Autodesk Inventor part; units mm, degrees
ref_plane "YZ Plane" through (0, 0, 0) normal (1, 0, 0) x (0, 1, 0)
ref_plane "XZ Plane" through (0, 0, 0) normal (0, 1, 0) x (-1, 0, 0)
ref_plane "XY Plane" through (0, 0, 0) normal (0, 0, 1) x (1, 0, 0)
sketch "스케치1" plane through (0, 0, 0) normal (0, 0, 1) x (1, 0, 0)
  line L0 (-350, 74) -> (350, 74)
  line L1 (350, 74) -> (350, -74)
  line L2 (350, -74) -> (-350, -74)
  line L3 (-350, -74) -> (-350, 74)
  line L4 (-340, 64.5) -> (-211.5, 64.5)
  line L5 (-211.5, 64.5) -> (-211.5, -64)
  line L6 (-211.5, -64) -> (-340, -64)
  line L7 (-340, -64) -> (-340, 64.5)
  line L8 (-201.5, 65) -> (-72.5, 65)
  line L9 (-72.5, 65) -> (-72.5, -64)
  line L10 (-72.5, -64) -> (-201.5, -64)
  line L11 (-201.5, -64) -> (-201.5, 65)
  line L12 (211, 65) -> (340, 65)
  line L13 (340, 65) -> (340, -64)
  line L14 (340, -64) -> (211, -64)
  line L15 (211, -64) -> (211, 65)
  line L16 (72.5, 64.5) -> (201, 64.5)
  line L17 (201, 64.5) -> (201, -64)
  line L18 (201, -64) -> (72.5, -64)
  line L19 (72.5, -64) -> (72.5, 64.5)
  circle A0 centre (0, 0) radius 50
  circle A1 centre (42.072, 42.072) radius 2
  circle A2 centre (-42.072, 42.072) radius 2
  circle A3 centre (-42.072, -42.072) radius 2
  circle A4 centre (42.072, -42.072) radius 2
  line L20 (-490, 0) -> (490, 0)
  line L21 (0, -103.6) -> (0, 103.6)
  point P0 (0, -74)
  point P1 (-72.5, 0.5)
  point P2 (-201.5, 0.5)
  point P3 (-137, -64)
  point P4 (-137, 65)
  point P5 (340, 0.5)
  point P6 (211, 0.5)
  point P7 (275.5, -64)
  point P8 (275.5, 65)
  point P9 (136.75, -64)
  point P10 (136.75, 64.5)
  point P11 (201, 0.25)
  point P12 (72.5, 0.25)
  dimension "d0" = 148
  dimension "d1" = 74
  dimension "d2" = 700
  dimension "d3" = 350
  dimension "d4" = 128.5
  dimension "d5" = 128.5
  dimension "d6" = 10
  dimension "d7" = 10
  dimension "d8" = 129
  dimension "d9" = 129
  dimension "d10" = 10
  dimension "d11" = 10
  dimension "d12" = 129
  dimension "d13" = 129
  dimension "d14" = 128.5
  dimension "d15" = 128.5
  dimension "d16" = 10
  dimension "d17" = 10
  dimension "d18" = 10
  dimension "d19" = 10
  dimension "d20" = 100
  dimension "d21" = 4
  dimension "d22" = 4
  dimension "d23" = 4
  dimension "d24" = 4
  dimension "d25" = 42.072
  dimension "d26" = 42.072
  dimension "d27" = 42.072
  dimension "d28" = 42.072
  dimension "d29" = 42.072
  dimension "d30" = 42.072
  dimension "d31" = 42.072
  dimension "d32" = 42.072
extrude "돌출3" add sketch "스케치1" along normal blind 2 contours L0 L21 A0 L20 L9 L8 L11 L5 L4 L7 L3 | L0 L1 L20 L13 L12 L15 L17 L16 L19 A0 L21 | L20 L7 L6 L5 L11 L10 L9 A0 L21 L2 L3 | L1 L2 L21 A0 L20 L19 L18 L17 L15 L14 L13
properties part number "가로로만"
Can you work these out from the model? Positions are in its coordinate system, mm. Coordinates: 2 decimals unless noted, no trailing zeros. Loops run counter-clockwise (first coordinate to the right, second up) from the corner with the lowest first, then second, coordinate; pieces in that order, holes last. Notation, with made-up numbers: M -33.75,48.5 L -2.75,48.5 A24 cw -2.75,75.5 Z; hole C 57,7 d4. An arc over 180 degrees is marked long. Answer as CSV lines item,"result". Start each with the question number.
1. Suppose I cut it at D-D, the plane z = 0.95. Count the separate pieces of the cut face and the enclosed holes in it, plus the area to 3 significant figures.
2. Suppose I cut it at A-A, the plane y = 0. List the corners of the cut face in (x, z) for me, plus the area to 3 significant figures.
3. Thinking about a two-plate mould opening in X: for faces 1 (the face through (-28, 44, 2)), 2 (the face through (47.69, -15.02, 0.99)), which applies, +X half, -X half, draft (parallel to the pull), parting line (faces both ways), or undercut?
4. Suppose I cut it at B-B, the plane x = -281. List the corners of the cut face in (y, z) for me.
5. For pin 1 Ø3.5 at (x, y) = (42.072, 42.072) entering from +Z, with a flat end and sliding along its axis, tell me the tip position at first contact or that it passes through.
6. Suppose I cut it at C-C, the plane x = 0. List the corners of the cut face in (y, z) for me.
7. If I drill on probe 1 along X at (y, z) = (50.5, 0.6); probe 2 along Y at (x, z) = (0, 1); probe 3 along X at (y, z) = (-8, 1.25), over which ranges is the centre line in solid material (lowest first)? Write a range as [from, to].
Output:
1,separate pieces,"1"
1,enclosed holes,"9"
1,area,"29,400 mm^2"
2,outline,"M -350,0 L -340,0 L -340,2 L -350,2 Z; M -211.5,0 L -201.5,0 L -201.5,2 L -211.5,2 Z; M -72.5,0 L -50,0 L -50,2 L -72.5,2 Z; M 50,0 L 72.5,0 L 72.5,2 L 50,2 Z; M 201,0 L 211,0 L 211,2 L 201,2 Z; M 340,0 L 350,0 L 350,2 L 340,2 Z"
2,area,"170 mm^2"
3,face 1,"draft"
3,face 2,"undercut"
4,outline,"M -74,0 L -64,0 L -64,2 L -74,2 Z; M 64.5,0 L 74,0 L 74,2 L 64.5,2 Z"
5,pin 1,"passes through"
6,outline,"M -74,0 L -50,0 L -50,2 L -74,2 Z; M 50,0 L 74,0 L 74,2 L 50,2 Z"
7,probe 1,"x = [-350, -340], [-211.5, -201.5], [-72.5, 72.5], [201, 211], [340, 350]"
7,probe 2,"y = [-74, -50], [50, 74]"
7,probe 3,"x = [-350, -340], [-211.5, -201.5], [-72.5, -49.36], [49.36, 72.5], [201, 211], [340, 350]"
